```python
from build123d import *

# Parameters (mm, degrees)
SKETCH_1_R           = 2.5
EXTRUDE_1_DEPTH      = 4.5
EXTRUDE_1_DEPTH_BACK = 4.5
SKETCH_3_R           = 0.5


with BuildPart() as part:
    # Sketch 1 → Extrude 1 (new body, two sides)
    with BuildSketch(Plane(origin=(0, 0, 0), x_dir=(0, 0, -1), z_dir=(1, 0, 0))) as extrude_1_sk:
        Circle(SKETCH_1_R)
    extrude(amount=EXTRUDE_1_DEPTH)
    extrude(extrude_1_sk.sketch, amount=-EXTRUDE_1_DEPTH_BACK)

    # Sweep 1: sweep along a path in Sketch 2
    with BuildLine(Plane.XY) as sweep_1_path:
        Line((7.62, -5.1), (7.62, -1))
        ThreePointArc((7.62, -1), (7.327106781, -0.292893219), (6.62, 0))
        Line((6.62, 0), (-6.62, 0))
        ThreePointArc((-6.62, 0), (-7.327106781, -0.292893219), (-7.62, -1))
        Line((-7.62, -1), (-7.62, -5.1))
    # Sketch 3 → Sweep 1 (sweep)
    with BuildSketch(Plane(origin=(4.5, 0, 0), x_dir=(0, 0, -1), z_dir=(1, 0, 0))):
        Circle(SKETCH_3_R)
    sweep(path=sweep_1_path.line)


solid = part.part
```
Design review of the part built by this model. Coordinates are the model's own, in mm. A direction names the side the tool comes from. Give positions to 0.01 mm unless a question says otherwise; leave off trailing zeros. Order: outer loops, then holes, each group sorted by start corner. A loop starts at its lowest first (then second) coordinate and runs counter-clockwise, first axis right, second up. Notation, with made-up numbers: (-36, 47.25) - (16, 47.25) arc R14 cw to (16, 66.25) - close; hole circle Ø5 at (79.5, -34.75). An arc over 180 degrees is marked (long way). Use a Markdown table: item, result. Add a question column.
(1) Machinability: for faces 4 (the face through (7.6, -5.1, 0)), 5 (the face through (-8.108, -3.079, 0.108)), 6 (the face through (5.545, 0.488, 0.108)), which of the approach directions +Z, -Z, +X, -X, +Y, -Y give a long, thin tool a straight path to every point of the face, cutting with its end or side? Answer none if there is none.
(2) Add section C-C on x = 2. Give the boundary of the cut face in (y, z).
(3) Wall thickness on probe 1 along X at (y, z) = (-2, -0.3); probe 2 along Y at (x, z) = (2.75, 0.1); probe 3 along X at (y, z) = (0.25, 1.25): over which ranges is each line inside the solid? List them lowest first. Write a range as [from, to].
(4) Mouldability with a two-part tool opening along X and no side actions: class faces 1 (the face through (8.108, -3.021, 0.108)), 2 (the face through (-7.6, -5.1, 0)), 3 (the face through (-5.575, 0.488, 0.108)) as +X half, -X half, draft (parallel to the pull), parting line (faces both ways), or undercut.
(5) Add section A-A on z = 0. Give the boundary of the cut face in (x, y).
(6) Add section D-D on y = -0.75. Give the number of separate pieces and of enclosed holes in the cut face, then the cut area to 3 significant figures.
(7) Add section B-B on y = -4.25. Give the boundary of the cut face in (x, z).
(8) Clearance check with flat-ended pins moving along their axes: P1, Ø1.5, axis at y = 0, z = -1, coming from the +X side; P2, Ø1, axis at y = 1.5, z = -1.5, coming from the +X side; P3, Ø1.5, axis at x = 3.5, y = -1, coming from the -Z side. State where each tip first meets the part, or that it passes through.
Report:
| question | item | result |
|---|---|---|
| 1 | face 4 | +Z, -Z, +X, -X, -Y |
| 1 | face 5 | -Y |
| 1 | face 6 | none |
| 2 | outline | circle Ø5 at (0, 0) |
| 3 | probe 1 | x = [-8.02, -7.22], [-4.5, 4.5], [7.22, 8.02] |
| 3 | probe 2 | y = [-2.5, 2.5] |
| 3 | probe 3 | x = [-4.5, 4.5] |
| 4 | face 1 | undercut |
| 4 | face 2 | draft |
| 4 | face 3 | undercut |
| 5 | outline | (-8.12, -5.1) - (-7.12, -5.1) - (-7.12, -1) arc R0.5 cw to (-6.62, -0.5) - (-4.5, -0.5) - (-4.5, -2.5) - (4.5, -2.5) - (4.5, -0.5) - (6.62, -0.5) arc R0.5 cw to (7.12, -1) - (7.12, -5.1) - (8.12, -5.1) - (8.12, -1) arc R1.5 ccw to (6.62, 0.5) - (4.5, 0.5) - (4.5, 2.5) - (-4.5, 2.5) - (-4.5, 0.5) - (-6.62, 0.5) arc R1.5 ccw to (-8.12, -1) - close |
| 6 | separate pieces | 3 |
| 6 | enclosed holes | 0 |
| 6 | area | 44.6 mm² |
| 7 | outline | circle Ø1 at (-7.62, 0); circle Ø1 at (7.62, 0) |
| 8 | P1 | stops at x = 7.83 |
| 8 | P2 | stops at x = 4.5 |
| 8 | P3 | stops at z = -2.49 |
